Autodesk Inventor part; units mm, degrees
ref_plane "YZ Plane" through (0, 0, 0) normal (1, 0, 0) x (0, 1, 0)
ref_plane "XZ Plane" through (0, 0, 0) normal (0, 1, 0) x (-1, 0, 0)
ref_plane "XY Plane" through (0, 0, 0) normal (0, 0, 1) x (1, 0, 0)
sketch "Szkic1" plane through (0, 0, 0) normal (0, 1, 0) x (-1, 0, 0)
  circle A0 centre (0, 0) radius 9.5
  circle A1 centre (0, 0) radius 25
  dimension "d0" = 19
  dimension "d3" = 50
extrude "Wyciągnięcie proste1" add sketch "Szkic1" along normal blind 7
sketch "Szkic2" plane through (0, 7, 0) normal (0, 1, 0) x (1, 0, 0)
  circle A0 centre (0, 0) radius 9.5
  circle A1 centre (0, 0) radius 8.5
  dimension "d4" = 19
  dimension "d5" = 17
extrude "Wyciągnięcie proste2" add sketch "Szkic2" against normal blind 1
chamfer "Faza1" distance 1 distance2 2 1 edges at (25, 0, 0) measured on face at (-24.9189, 4.6667, -2.0117)
properties part number "opona_nosne" material "Aluminum 6061"
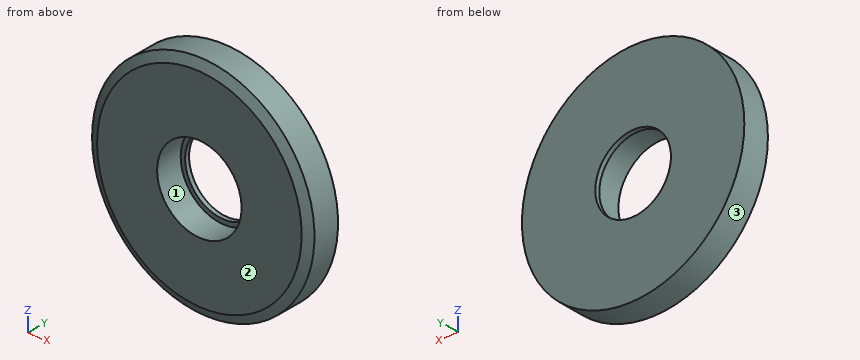
The listing builds one solid part. Answer for the finished solid, in the listing's coordinates (mm). Face numbers are marked on the shaded views. Give positions to 0.01 mm unless a question says otherwise; leave off trailing zeros. Loops run counter-clockwise (first coordinate to the right, second up) from the corner with the lowest first, then second, coordinate; pieces in that order, holes last. Notation, with made-up numbers: (-34.5, 80.5) - (2.5, 80.5) arc R21 cw to (2.5, 104.5) - close; hole circle Ø8 at (76.5, 41.25). An arc over 180 degrees is marked (long way). Answer as CSV lines item,"result". Start each with the question number.
Item 1: A cutting plane is placed at C-C on y = 4.5. Determine the outline of the cut face in (x, z).
Item 2: A cutting plane is placed at B-B on x = 0. Determine the outline of the cut face in (y, z), then the cut area to 3 significant figures.
Item 3: A cutting plane is placed at A-A on z = 0. Determine the outline of the cut face in (x, y).
Item 4: Find the intervals of material crossed by line 1 (Z direction, x = 0, y = 2.65); line 2 (Z direction, x = 0, y = 6.7); line 3 (X direction, y = 0.75, z = -5), in increasing order. Write a range as from..to.
Item 5: The mould has two halves that part along Z. Classify the marked faces 1, 2 and 3: +Z half, -Z half, draft (parallel to the pull), parting line (faces both ways), or undercut.
Item 6: Each of these flat-tipped pins is pushed along its axis until it touches: pin 1 (1.5 mm diameter, centred on x = -16.5, y = 3.5, fed in from -Z); pin 2 (2 mm diameter, centred on y = 3.5, z = -12.5, fed in from -X); pin 3 (4 mm diameter, centred on x = 17.5, y = 1, fed in from -Z). Where does it stop, or does it pass through?
Found:
1,outline,"circle Ø50 at (0, 0); hole circle Ø19 at (0, 0)"
2,outline,"(0, -23) - (1, -25) - (7, -25) - (7, -8.5) - (6, -8.5) - (6, -9.5) - (0, -9.5) - close; (0, 9.5) - (6, 9.5) - (6, 8.5) - (7, 8.5) - (7, 25) - (1, 25) - (0, 23) - close"
2,area,"217 mm^2"
3,outline,"(-25, 1) - (-23, 0) - (-9.5, 0) - (-9.5, 6) - (-8.5, 6) - (-8.5, 7) - (-25, 7) - close; (8.5, 6) - (9.5, 6) - (9.5, 0) - (23, 0) - (25, 1) - (25, 7) - (8.5, 7) - close"
4,line 1,"z = -25..-9.5, 9.5..25"
4,line 2,"z = -25..-8.5, 8.5..25"
4,line 3,"x = -23.98..-8.08, 8.08..23.98"
5,face 1,"undercut"
5,face 2,"draft"
5,face 3,"parting line"
6,pin 1,"stops at z = -19.41"
6,pin 2,"stops at x = -22.2"
6,pin 3,"stops at z = -19.62"
